Autodesk Inventor part; units mm, degrees
ref_plane "YZ Plane" through (0, 0, 0) normal (1, 0, 0) x (0, 1, 0)
ref_plane "XZ Plane" through (0, 0, 0) normal (0, 1, 0) x (-1, 0, 0)
ref_plane "XY Plane" through (0, 0, 0) normal (0, 0, 1) x (1, 0, 0)
sketch "Sketch1" plane through (0, 0, 0) normal (0, 1, 0) x (-1, 0, 0)
  line L0 (34, 34) -> (-34, 34)
  line L1 (-34, 34) -> (-34, -34)
  line L2 (-34, -34) -> (34, -34)
  line L3 (34, -34) -> (34, 34)
  line L4 (34, 34) -> (-34, -34) construction
  line L5 (-34, 34) -> (34, -34) construction
  point P0 (0, 0)
  dimension "d0" = 68
  dimension "d1" = 68
extrude "Extrusion1" add sketch "Sketch1" along normal blind 1
sketch "Sketch2" plane through (0, 1, 0) normal (0, 1, 0) x (1, 0, 0)
  line L0 (34, -34) -> (34, 34)
  line L1 (34, 34) -> (-34, 34)
  line L2 (-34, 34) -> (-34, -34)
  line L3 (-34, -34) -> (34, -34)
  line L4 (-32.4, -32.4) -> (-32.4, 32.4)
  line L5 (-32.4, 32.4) -> (32.4, 32.4)
  line L6 (32.4, 32.4) -> (32.4, -32.4)
  line L7 (32.4, -32.4) -> (-32.4, -32.4)
  point P0 (0, 0)
  dimension "d4" = 1.6
extrude "Extrusion2" add sketch "Sketch2" along normal blind 26
fillet "Fillet1" radius 3.5 4 edges at (-32.4, 14, 32.4) (-32.4, 14, -32.4) (32.4, 14, -32.4) (32.4, 14, 32.4)
fillet "Fillet2" radius 5.5 4 edges at (34, 13.5, 34) (34, 13.5, -34) (-34, 13.5, -34) (-34, 13.5, 34)
fillet "Fillet3" radius 2 8 edges at (-31.3749, 1, 31.3749) (0, 1, 32.4) (31.3749, 1, 31.3749) (32.4, 1, 0) (31.3749, 1, -31.3749) (0, 1, -32.4) (-31.3749, 1, -31.3749) (-32.4, 1, 0)
fillet "Fillet4" radius 3 8 edges at (-32.3891, 0, 32.3891) (0, 0, 34) (32.3891, 0, 32.3891) (34, 0, 0) (32.3891, 0, -32.3891) (0, 0, -34) (-32.3891, 0, -32.3891) (-34, 0, 0)
sketch "Sketch3" plane through (0, 27, 0) normal (0, 1, 0) x (1, 0, 0)
  arc A0 (-34, -28.5) -> (-28.5, -34) centre (-28.5, -28.5) ccw
  line L0 (-28.5, -34) -> (28.5, -34)
  arc A1 (28.5, -34) -> (34, -28.5) centre (28.5, -28.5) ccw
  line L1 (34, -28.5) -> (34, 28.5)
  arc A2 (34, 28.5) -> (28.5, 34) centre (28.5, 28.5) ccw
  line L2 (28.5, 34) -> (-28.5, 34)
  arc A3 (-28.5, 34) -> (-34, 28.5) centre (-28.5, 28.5) ccw
  line L3 (-34, 28.5) -> (-34, -28.5)
  line L4 (-32.4, -28.9) -> (-32.4, 28.9)
  arc A4 (-28.9, 32.4) -> (-32.4, 28.9) centre (-28.9, 28.9) ccw
  line L5 (-28.9, 32.4) -> (28.9, 32.4)
  arc A5 (32.4, 28.9) -> (28.9, 32.4) centre (28.9, 28.9) ccw
  line L6 (32.4, 28.9) -> (32.4, -28.9)
  arc A6 (28.9, -32.4) -> (32.4, -28.9) centre (28.9, -28.9) ccw
  line L7 (28.9, -32.4) -> (-28.9, -32.4)
  arc A7 (-32.4, -28.9) -> (-28.9, -32.4) centre (-28.9, -28.9) ccw
  line L8 (-34, 28.5) -> (-34, -28.5)
  line L9 (-34, 0) -> (34, 0)
  line L10 (34, -28.5) -> (34, 28.5)
  line L11 (-28.5, -34) -> (28.5, -34)
  line L12 (0, -34) -> (0, 34)
  line L13 (-0.6, -34) -> (-0.6, 34)
  line L14 (0.6, -34) -> (0.6, 34)
  line L15 (-34, 0.6) -> (34, 0.6)
  line L16 (-34, -0.6) -> (34, -0.6)
  point P0 (0, 0)
  point P1 (-0.6, 0.6)
  point P2 (-32.4, 0.6)
  point P3 (-32.4, -0.6)
  point P4 (-0.6, -0.6)
  point P5 (-0.6, -32.4)
  point P6 (0.6, -32.4)
  point P7 (0.6, -0.6)
  point P8 (32.4, -0.6)
  point P9 (32.4, 0.6)
  point P10 (0.6, 0.6)
  point P11 (0.6, 32.4)
  point P12 (-0.6, 32.4)
  dimension "d11" = 0.6
  dimension "d12" = 0.6
  dimension "d13" = 0.6
  dimension "d14" = 0.6
extrude "Extrusion3" add sketch "Sketch3" against normal up to surface (26 mm away) contours L4 L9 L13 L16 | L13 L16 L12 L7 | L4 L15 L13 L9 | L13 L9 L12 L16 | L12 L16 L14 L7 | L13 L15 L12 L9 | L12 L9 L14 L16 | L13 L5 L12 L15 | L12 L15 L14 L9 | L14 L9 L6 L16 | L12 L5 L14 L15 | L14 L15 L6 L9
fillet "Fillet5" radius 1 4 edges at (0.6, 14, 0.6) (-0.6, 14, 0.6) (0.6, 14, -0.6) (-0.6, 14, -0.6)
fillet "Fillet6" radius 1 28 edges at (0.6, 1.5858, 31.8142) (0.6, 1, 16) (0.8929, 1, 0.8929) (16, 1, 0.6) (31.8142, 1.5858, 0.6) (32.4, 15, 0.6) (0.6, 15, 32.4) (31.8142, 1.5858, -0.6) (32.4, 15, -0.6) (0.8929, 1, -0.8929) (0.6, 1, -16) (0.6, 1.5858, -31.8142) (0.6, 15, -32.4) (16, 1, -0.6) (-0.8929, 1, -0.8929) (-0.6, 1, -16) (-0.6, 1.5858, -31.8142) (-0.6, 15, -32.4) (-31.8142, 1.5858, -0.6) (-32.4, 15, -0.6) (-16, 1, -0.6) (-31.8142, 1.5858, 0.6) (-32.4, 15, 0.6) (-0.8929, 1, 0.8929) (-0.6, 1, 16) (-0.6, 1.5858, 31.8142) (-0.6, 15, 32.4) (-16, 1, 0.6)
The listing builds one solid part. Answer for the finished solid, in the listing's coordinates (mm). A direction names the side the tool comes from. Round coordinates to 2 decimals unless told otherwise and drop trailing zeros. Order: outer loops, then holes, each group sorted by start corner. A loop starts at its lowest first (then second) coordinate and runs counter-clockwise, first axis right, second up. Notation, with made-up numbers: (83, 76) - (137, 76) arc R30 ccw to (137, 110) - close; hole circle Ø6 at (-36, -11.5). An arc over 180 degrees is marked (long way). Put each result on its own line as item: value. Start each with the question number.
(1) For faces 4 (the cylindrical face through (-33.1, 0.86, -0.4)), 5 (the flat face through (-32.4, 15, 15)), determine the directions among +Z, -Z, +X, -X, +Y, -Y from which every point of the face is accessible in a straight line to the end or side of a thin tool.
(2) Given P1, Ø8, axis at x = -22, z = 18, coming from the +Y side; P2, Ø23, axis at x = 22.5, z = -20.5, coming from the +Y side, each flat-ended and moving along its own axis, determine where each tip first touches the part or whether it passes through.
(3) Determine the mould class of faces 1 (the cylindrical face through (0.4, 0.86, -33.1)), 2 (the cylindrical face through (-32.43, 15.17, 32.35)), 3 (the cylindrical face through (31.8, 1.57, -15.06)) for opening direction X: released by +X, released by -X, zero draft, split by the parting line, or undercut.
(4) Find section C-C (x = -9.5). Give the vertices of the cut face in (y, z).
(5) Find section A-A (z = -19.5). Give the vertices of the cut face in (x, y), plus the area to 3 significant figures.
(6) Straight lines are drawn through the part: probe 1 along X at (y, z) = (6.75, -2); probe 2 along Y at (x, z) = (4, -24.5). For each, find the intervals that lie inside material, in ascending order. Write a range as from..to.
(7) Find section B-B (y = 7.5). State how many separate pieces and enclosed holes the cut face has, plus the area to 3 significant figures.
Reply:
1. face 4: +Z, -Z, -X, -Y
1. face 5: +Y
2. P1: y = 1
2. P2: y = 27
3. face 1: zero draft
3. face 2: released by -X
3. face 3: undercut
4. outline: (0, -31) arc R3 ccw to (3, -34) - (27, -34) - (27, -32.4) - (3, -32.4) arc R2 cw to (1, -30.4) - (1, -1.6) arc R1 cw to (2, -0.6) - (27, -0.6) - (27, 0.6) - (2, 0.6) arc R1 cw to (1, 1.6) - (1, 30.4) arc R2 cw to (3, 32.4) - (27, 32.4) - (27, 34) - (3, 34) arc R3 ccw to (0, 31) - close
5. outline: (-34, 3) arc R3 ccw to (-31, 0) - (31, 0) arc R3 ccw to (34, 3) - (34, 27) - (32.4, 27) - (32.4, 3) arc R2 cw to (30.4, 1) - (1.6, 1) arc R1 cw to (0.6, 2) - (0.6, 27) - (-0.6, 27) - (-0.6, 2) arc R1 cw to (-1.6, 1) - (-30.4, 1) arc R2 cw to (-32.4, 3) - (-32.4, 27) - (-34, 27) - close
5. area: 181 mm^2
6. probe 1: -34..-32.4, -0.6..0.6, 32.4..34
6. probe 2: 0..1
7. separate pieces: 1
7. enclosed holes: 4
7. area: 566 mm^2
